```python
from build123d import *

# Parameters (mm, degrees)
BOSS_EXTRUDE1_DEPTH = 1.4
BOSS_EXTRUDE2_DEPTH = 15
SKETCH6_W           = 17
SKETCH6_H           = 17
BOSS_EXTRUDE3_DEPTH = 6
CUT_EXTRUDE4_START  = -16
SKETCH8_W           = 17
SKETCH8_H           = 7
CUT_EXTRUDE4_DEPTH  = 16
SKETCH9_W           = 17
SKETCH9_H           = 22.4
BOSS_EXTRUDE4_DEPTH = 2
SKETCH7_4_R         = 2.45
CUT_EXTRUDE3_DEPTH  = 4.5
CHAMFER1_SIZE       = 4
CHAMFER3_SIZE       = 4
CUT_EXTRUDE5_REACH  = 28.158
CHAMFER4_SIZE       = 1
SPLIT1_START        = 2.45
SPLIT1_DEPTH        = 4.05
SPLIT1_START_2      = -4.5
SPLIT1_2_DEPTH      = 2.0499999
SPLIT1_START_3      = -21
SPLIT1_3_DEPTH      = 6
SPLIT1_START_4      = -16.5
SPLIT1_4_OUTLINE_R  = 2.45
SPLIT1_4_DEPTH      = 1.5
SPLIT1_START_5      = -20.859650045
SPLIT1_5_OUTLINE_W  = 20
SPLIT1_5_OUTLINE_H  = 18
SPLIT1_5_DEPTH      = 2.828427125
SPLIT1_START_6      = -22.273863607
SPLIT1_6_OUTLINE_W  = 20
SPLIT1_6_OUTLINE_H  = 18
SPLIT1_6_DEPTH      = 2.828427124
SPLIT1_START_7      = -9
SPLIT1_7_DEPTH      = 20
SPLIT1_8_DEPTH      = 14


with BuildPart() as part:
    # Sketch3 → Boss-Extrude1 (new body)
    with BuildSketch(Plane(origin=(0, 0, 0), x_dir=(1, 0, 0), z_dir=(0, 1, 0))):
        with BuildLine():
            Line((-3.15, 0), (-3.15, 8.5))
            Line((-3.15, 8.5), (-8.5, 8.5))
            Line((-8.5, 8.5), (-8.5, -8.5))
            Line((-8.5, -8.5), (8.5, -8.5))
            Line((8.5, -8.5), (8.5, 8.5))
            Line((8.5, 8.5), (3.15, 8.5))
            Line((3.15, 8.5), (3.15, 0))
            ThreePointArc((3.15, 0), (0, -3.15), (-3.15, 0))
        make_face()
    extrude(amount=BOSS_EXTRUDE1_DEPTH)

    # Sketch4 → Boss-Extrude2 (add)
    with BuildSketch(Plane.XZ):
        with BuildLine():
            Line((7.5, 0), (7.5, -8.5))
            Line((7.5, -8.5), (8.5, -8.5))
            Line((8.5, -8.5), (8.5, 8.5))
            Line((8.5, 8.5), (-8.5, 8.5))
            Line((-8.5, 8.5), (-8.5, -8.5))
            Line((-8.5, -8.5), (-7.5, -8.5))
            Line((-7.5, -8.5), (-7.5, 0))
            ThreePointArc((-7.5, 0), (0, 7.5), (7.5, 0))
        make_face()
    extrude(amount=BOSS_EXTRUDE2_DEPTH)

    # Sketch6 → Boss-Extrude3 (add)
    with BuildSketch(Plane.XZ.offset(15)):
        Rectangle(SKETCH6_W, SKETCH6_H)
    extrude(amount=BOSS_EXTRUDE3_DEPTH)

    # Sketch8 → Cut-Extrude4 (cut)
    with BuildSketch(Plane(origin=(0, 0, -8.5), x_dir=(-1, 0, 0), z_dir=(0, 0, -1)).offset(CUT_EXTRUDE4_START)):
        with Locations((0, -3.5)):
            Rectangle(SKETCH8_W, SKETCH8_H)
    extrude(amount=CUT_EXTRUDE4_DEPTH, mode=Mode.SUBTRACT)

    # Sketch9 → Boss-Extrude4 (add)
    with BuildSketch(Plane.XY.offset(8.5)):
        with Locations((0, -9.8)):
            Rectangle(SKETCH9_W, SKETCH9_H)
    extrude(amount=BOSS_EXTRUDE4_DEPTH)

    # Sketch7<4> → Cut-Extrude3 (cut)
    with BuildSketch(Plane.XZ.offset(21)):
        with Locations(Location((0, 0, 0), (0, 0, 270))):
            Circle(SKETCH7_4_R)
    extrude(amount=-CUT_EXTRUDE3_DEPTH, mode=Mode.SUBTRACT)

    # Chamfer1
    chamfer1_edges = [part.edges().sort_by_distance(p)[0] for p in [
        (0, -21, 10.5),
        (-8.5, -21, 1),
        (0, -21, -8.5),
        (8.5, -21, 1),
    ]]
    chamfer(chamfer1_edges, length=CHAMFER1_SIZE)

    # Chamfer3
    # the kernel refuses this chamfer: 4 mm, written as the material it takes off along each edge
    with BuildSketch(Plane(origin=(8.5, -27.286731952, 10.5), x_dir=(-1, 0, 0), z_dir=(0, 1, 0))) as chamfer3_piece_1:
        Polygon((CHAMFER3_SIZE, 0), (0, -CHAMFER3_SIZE), (0, 0), align=None)
    extrude(amount=38.973463904, mode=Mode.SUBTRACT)
    with BuildSketch(Plane(origin=(8.5, -7, -8.5), x_dir=(-1, 0, 0), z_dir=(0, -1, 0))) as chamfer3_piece_2:
        Polygon((CHAMFER3_SIZE, 0), (0, -CHAMFER3_SIZE), (0, 0), align=None)
    extrude(amount=20.286731952, mode=Mode.SUBTRACT)
    with BuildSketch(Plane(origin=(-8.5, -27.286731952, -8.5), x_dir=(0, 0, 1), z_dir=(0, 1, 0))) as chamfer3_piece_3_section:
        Polygon((CHAMFER3_SIZE, 0), (0, CHAMFER3_SIZE), (0, 0), align=None)
    chamfer3_piece_3 = extrude(amount=30.573463904, mode=Mode.PRIVATE)
    chamfer3_piece_3 = split(chamfer3_piece_3, bisect_by=Plane(origin=(-8.5, 0, -8.5), z_dir=(0, -1, 0)), keep=Keep.TOP, mode=Mode.PRIVATE)
    add(chamfer3_piece_3, mode=Mode.SUBTRACT)
    with BuildSketch(Plane(origin=(-8.5, 11.686731952, 10.5), x_dir=(0, 0, -1), z_dir=(0, -1, 0))) as chamfer3_piece_4:
        Polygon((CHAMFER3_SIZE, 0), (0, CHAMFER3_SIZE), (0, 0), align=None)
    extrude(amount=38.973463904, mode=Mode.SUBTRACT)

    # Sketch10 → Cut-Extrude5 (cut, up to next)
    with BuildSketch(Plane(origin=(0, 1.4, 0), x_dir=(1, 0, 0), z_dir=(0, 1, 0)), mode=Mode.PRIVATE) as cut_extrude5_sk1:
        Polygon((7.5, -7.5), (7.5, 8.5), (8.5, 8.5), (8.5, -6.5), align=None)
    cut_extrude5_tool1 = extrude(cut_extrude5_sk1.sketch, amount=-CUT_EXTRUDE5_REACH, mode=Mode.PRIVATE) & part.part
    # Sketch10 → Cut-Extrude5 (cut, up to next)
    with BuildSketch(Plane(origin=(0, 1.4, 0), x_dir=(1, 0, 0), z_dir=(0, 1, 0)), mode=Mode.PRIVATE) as cut_extrude5_sk2:
        Polygon((-7.5, -7.5), (-7.5, 8.5), (-8.5, 8.5), (-8.5, -6.5), align=None)
    cut_extrude5_tool2 = extrude(cut_extrude5_sk2.sketch, amount=-CUT_EXTRUDE5_REACH, mode=Mode.PRIVATE) & part.part
    add(cut_extrude5_tool1.solids().sort_by_distance((7.994624, 1.4, -0.747312))[0], mode=Mode.SUBTRACT)
    add(cut_extrude5_tool2.solids().sort_by_distance((-7.994624, 1.4, -0.747312))[0], mode=Mode.SUBTRACT)

    # Chamfer4
    chamfer4_edges = [part.edges().sort_by_distance(p)[0] for p in [
        (7.5, 0.7, -8.5),
        (-7.5, 0.7, -8.5),
    ]]
    chamfer(chamfer4_edges, length=CHAMFER4_SIZE)

    # Split1 8 outline → Split1 8 (cut)
    with BuildSketch(Plane(origin=(0, 0, 0), x_dir=(1, 0, 0), z_dir=(0, 1, 0)).offset(SPLIT1_START_3)):
        Polygon((-8.5, 4.5), (-8.5, -6.5), (-4.5, -10.5), (4.5, -10.5), (8.5, -6.5), (8.5, 4.5), (4.5, 8.5), (-4.5, 8.5), align=None)
    extrude(amount=SPLIT1_8_DEPTH, mode=Mode.SUBTRACT)


with BuildPart() as body_2:
    # Split1: read off the stored shape, not the designer's step
    # Split1 outline → Split1 (new body)
    with BuildSketch(Plane.XY.offset(SPLIT1_START)):
        Polygon((8.5, -17), (8.5, -15), (-8.5, -15), (-8.5, -17), (-4.5, -21), (4.5, -21), align=None)
    extrude(amount=SPLIT1_DEPTH)

    # Split1 2 outline → Split1 2 (add)
    with BuildSketch(Plane.XY.offset(SPLIT1_START_2)):
        Polygon((8.5, -17), (8.5, -15), (-8.5, -15), (-8.5, -17), (-4.5, -21), (4.5, -21), align=None)
    extrude(amount=SPLIT1_2_DEPTH)

    # Split1 3 outline → Split1 3 (add)
    with BuildSketch(Plane(origin=(0, 0, 0), x_dir=(1, 0, 0), z_dir=(0, 1, 0)).offset(SPLIT1_START_3)):
        with BuildLine():
            ThreePointArc((0, 2.45), (2.45, 0), (0, -2.45))
            Line((0, -2.45), (8.5, -2.45))
            Line((8.5, -2.45), (8.5, 2.4500001))
            Line((8.5, 2.4500001), (0, 2.45))
        make_face()
        with BuildLine():
            ThreePointArc((0, -2.45), (-2.45, 0), (0, 2.45))
            Line((0, 2.45), (-8.5, 2.4500001))
            Line((-8.5, 2.4500001), (-8.5, -2.45))
            Line((-8.5, -2.45), (0, -2.45))
        make_face()
        Polygon((-4.5, 8.5), (-8.5, 4.5), (8.5, 4.5), (4.5, 8.5), align=None)
        Polygon((8.5, -6.5), (-8.5, -6.5), (-4.5, -10.5), (4.5, -10.5), align=None)
    extrude(amount=SPLIT1_3_DEPTH)

    # Split1 4 outline → Split1 4 (add)
    with BuildSketch(Plane(origin=(0, 0, 0), x_dir=(1, 0, 0), z_dir=(0, 1, 0)).offset(SPLIT1_START_4)):
        Circle(SPLIT1_4_OUTLINE_R)
    extrude(amount=SPLIT1_4_DEPTH)

    # Split1 5 outline → Split1 5 (cut)
    with BuildSketch(Plane(origin=(0, 0, 0), x_dir=(1, 0, 0), z_dir=(0, 0.707106781186546, 0.707106781186549)).offset(SPLIT1_START_5)):
        with Locations((0, -14)):
            Rectangle(SPLIT1_5_OUTLINE_W, SPLIT1_5_OUTLINE_H)
    extrude(amount=SPLIT1_5_DEPTH, mode=Mode.SUBTRACT)

    # Split1 6 outline → Split1 6 (cut)
    with BuildSketch(Plane(origin=(0, 0, 0), x_dir=(1, 0, 0), z_dir=(0, 0.707106781186546, -0.707106781186549)).offset(SPLIT1_START_6)):
        with Locations((0, 12)):
            Rectangle(SPLIT1_6_OUTLINE_W, SPLIT1_6_OUTLINE_H)
    extrude(amount=SPLIT1_6_DEPTH, mode=Mode.SUBTRACT)

    # Split1 7 outline → Split1 7 (cut)
    with BuildSketch(Plane.XY.offset(SPLIT1_START_7)):
        Polygon((-8.5, -21), (-4.5, -21), (-8.5, -17), align=None)
        Polygon((8.5, -21), (8.5, -17), (4.5, -21), align=None)
    extrude(amount=SPLIT1_7_DEPTH, mode=Mode.SUBTRACT)


with BuildPart() as body_2_1:
    # Body-Move/Copy2: read off the stored shape, not the designer's step
    # Body-Move/Copy2: moved
    add(body_2.part.moved(Location((0, 8, 0))))


with BuildPart() as part_1:
    add(part.part)

    # Combine2: union body 2
    add(body_2_1.part)


solid = part_1.part
```
The listing builds one solid part. Answer for the finished solid, in the listing's coordinates (mm). A direction names the side the tool comes from. Give positions to 0.01 mm unless a question says otherwise; leave off trailing zeros. Loops run counter-clockwise (first coordinate to the right, second up) from the corner with the lowest first, then second, coordinate; pieces in that order, holes last. Notation, with made-up numbers: (15, 27.25) - (54, 27.25) arc R21 ccw to (54, 62.25) - close; hole circle Ø11 at (-34.5, 57.5). An arc over 180 degrees is marked (long way). Answer as CSV lines item,"result". Start each with the question number.
Item 1: A cutting plane is placed at A-A on y = -10.25. Determine the outline of the cut face in (x, z).
Item 2: A cutting plane is placed at C-C on x = 5. Determine the outline of the cut face in (y, z), then the cut area to 3 significant figures.
Item 3: For faces 1 (the face through (7.5, 1, 0)), 2 (the face through (-3.15, 1, -4)), 3 (the face through (0, -8.5, 0)), determine the directions among +Z, -Z, +X, -X, +Y, -Y from which every point of the face is accessible in a straight line to the end or side of a thin tool.
Item 4: Find the intervals of material crossed by line 1 (Y direction, x = 1.25, z = -2.75); line 2 (Y direction, x = -6, z = -6.5); line 3 (Y direction, x = -1.25, z = 5.5), in increasing order. Write a range as from..to.
Item 5: The mould has two halves that part along Z. Classify faces 4 (the face through (-0.938, -10.782, -2.263)), 5 (the face through (-0.1, -11, 8.5)), 6 (the face through (3.15, 1, -4)): +Z half, -Z half, draft (parallel to the pull), parting line (faces both ways), or undercut.
Item 6: A cutting plane is placed at D-D on z = -0.75. Determine the outline of the cut face in (x, y).
Item 7: A cutting plane is placed at B-B on z = 4. Determine the outline of the cut face in (x, y).
Item 8: Each of these flat-tipped pins is pushed along its axis until it touches: pin 1 (6.5 mm diameter, centred on x = 0, z = 0, fed in from -Y); pin 2 (0.7 mm diameter, centred on y = 1, z = -2.5, fed in from -X); pin 3 (1.1 mm diameter, centred on y = 1, z = 1.5, fed in from +X); pin 4 (1.5 mm diameter, centred on x = 1, z = 1, fed in from -Y). Where does it stop, or does it pass through?
Found:
1,outline,"(-7.25, -5.75) - (-5.75, -7.25) - (5.75, -7.25) - (7.25, -5.75) - (7.25, 7.75) - (5.75, 9.25) - (-5.75, 9.25) - (-7.25, 7.75) - close; hole circle Ø4.9 at (0, 0)"
2,outline,"(-12.5, -5) - (-9.5, -8) - (-7, -8) - (-7, 7.5) - (0, 7.5) - (0, -8.5) - (1.4, -8.5) - (1.4, 10) - (-9.5, 10) - (-12.5, 7) - close"
2,area,"133 mm^2"
3,face 1,"+Z, -Z, +X, +Y"
3,face 2,"-Z, +Y"
3,face 3,"-Y"
4,line 1,"y = -13..-7"
4,line 2,"y = -11..-7, 0..1.4"
4,line 3,"y = -13..-7, 0..1.4"
5,face 4,"undercut"
5,face 5,"+Z half"
5,face 6,"draft"
6,outline,"(-8.5, -9) - (-4.5, -13) - (-2.33, -13) - (-2.33, -8.5) - (2.33, -8.5) - (2.33, -13) - (4.5, -13) - (8.5, -9) - (8.5, -7) - (-8.5, -7) - close; (-7.5, 0) - (-3.15, 0) - (-3.15, 1.4) - (-7.5, 1.4) - close; (3.15, 0) - (7.5, 0) - (7.5, 1.4) - (3.15, 1.4) - close"
7,outline,"(-8.5, -9) - (-4.5, -13) - (4.5, -13) - (8.5, -9) - (8.5, -7) - (-8.5, -7) - close; (-7.5, 0) - (7.5, 0) - (7.5, 1.4) - (-7.5, 1.4) - close"
8,pin 1,"stops at y = -13"
8,pin 2,"stops at x = -7.5"
8,pin 3,"stops at x = 7.5"
8,pin 4,"stops at y = -8.5"
